Work out the finished part from the listing and answer in its coordinate system (mm). A direction names the side the tool comes from. Coordinates: 2 decimals unless noted, no trailing zeros. Order: outer loops, then holes, each group sorted by start corner. A loop starts at its lowest first (then second) coordinate and runs counter-clockwise, first axis right, second up. Notation, with made-up numbers: M -39,82 L -35,82 A23 cw -35,101 Z; hole C 46.5,1.5 d3. An arc over 180 degrees is marked long. Write item = value, one per line. Start each with the question number.
Q1. Find section C-C on x = 67.5. Give the vertices of the cut face in (y, z).
Q2. Find section A-A on x = -177. Give the vertices of the cut face in (y, z), and give its area (3 significant figures).
Q3. A tool of negligible diameter and unlimited length cuts with its end or side. For faces 4 (the flat face through (7, 0, 2)), 5 (the flat face through (0, 15, 147)), from which of +Z, -Z, +X, -X, +Y, -Y can it reach the whole face along a straight path? Write none if from no direction.
Q4. Determine the mould class of faces 1 (the flat face through (-500, 15, -13)), 2 (the cylindrical face through (7, 18.755, -171.923)), 3 (the flat face through (-253, 15, 145)) for opening direction Z: released by +Z, released by -Z, zero draft, split by the parting line, or undercut.
Q5. Find section B-B on y = 15. Give the vertices of the cut face in (x, z), and give its area (4 significant figures).
Q6. Straight lines are drawn through the part: line 1 along Z through (x, y) = (271, 19.5); line 2 along Z through (x, y) = (-10, 13.5); line 3 along Z through (x, y) = (262.5, 6). For each, find the intervals that lie inside material, in ascending order.
Q7. Each of these flat-tipped pins is pushed along its axis until it touches: P1, Ø12, axis at x = -247, y = 12, coming from the +Z side; P2, Ø12, axis at x = -304, y = 8, coming from the -Z side. Where does it stop, or does it pass through?
```python
from build123d import *

# Parameters (mm, degrees)
SKETCH1_W           = 1000
SKETCH1_H           = 290
BOSS_EXTRUDE1_DEPTH = 30
SKETCH2_R           = 15
SKETCH2_R_2         = 12.5
BOSS_EXTRUDE2_DEPTH = 500
SKETCH3_R           = 15
SKETCH3_R_2         = 12.5
BOSS_EXTRUDE3_DEPTH = 1000


with BuildPart() as part:
    # Sketch1 → Boss-Extrude1 (new body)
    with BuildSketch(Plane(origin=(0, 0, 0), x_dir=(1, 0, 0), z_dir=(0, 1, 0))):
        Rectangle(SKETCH1_W, SKETCH1_H)
    extrude(amount=BOSS_EXTRUDE1_DEPTH)

    # Sketch2 → Boss-Extrude2 (add)
    with BuildSketch(Plane(origin=(500, 0, 0), x_dir=(0, 0, -1), z_dir=(1, 0, 0))):
        with BuildLine():
            Line((-145, 30), (-160, 30))
            ThreePointArc((-160, 30), (-149.393398282, 25.606601718), (-145, 15))
            Line((-145, 15), (-145, 30))
        make_face()
        with BuildLine():
            Line((-145, 0), (-145, 15))
            ThreePointArc((-145, 15), (-149.393398282, 4.393398282), (-160, 0))
            Line((-160, 0), (-145, 0))
        make_face()
        with Locations((-160, 15)):
            Circle(SKETCH2_R)
        with Locations((-160, 15)):
            Circle(SKETCH2_R_2, mode=Mode.SUBTRACT)
    extrude(amount=-BOSS_EXTRUDE2_DEPTH)

    # Sketch3 → Boss-Extrude3 (add)
    with BuildSketch(Plane(origin=(500, 0, 0), x_dir=(0, 0, -1), z_dir=(1, 0, 0))):
        with BuildLine():
            ThreePointArc((145, 15), (149.393398282, 25.606601718), (160, 30))
            Line((160, 30), (145, 30))
            Line((145, 30), (145, 15))
        make_face()
        with Locations((160, 15)):
            Circle(SKETCH3_R)
        with Locations((160, 15)):
            Circle(SKETCH3_R_2, mode=Mode.SUBTRACT)
        with BuildLine():
            ThreePointArc((160, 0), (149.393398282, 4.393398282), (145, 15))
            Line((145, 15), (145, 0))
            Line((145, 0), (160, 0))
        make_face()
    extrude(amount=-BOSS_EXTRUDE3_DEPTH)


solid = part.part
```
Findings below:
q1.outline = M 0,-160 A15 ccw 30,-160 L 30,160 A15 ccw 0,160 Z; hole C 15,-160 d25; hole C 15,160 d25
q2.outline = M 0,-160 A15 ccw 30,-160 L 30,145 L 0,145 Z; hole C 15,-160 d25
q2.area = 9,010 mm^2
q3.face_4 = +Z, -Z, +X, -X, -Y
q3.face_5 = +Z, -X, +Y, -Y
q4.face_1 = zero draft
q4.face_2 = undercut
q4.face_3 = released by +Z
q5.outline = M -500,-175 L 500,-175 L 500,-172.5 L -500,-172.5 Z; M -500,-147.5 L 500,-147.5 L 500,147.5 L 0,147.5 L 0,145 L -500,145 Z; M 0,172.5 L 500,172.5 L 500,175 L 0,175 Z
q5.area = 297,500 mm^2
q6.line_1 = -174.31 to -171.66, -148.34 to 148.34, 171.66 to 174.31
q6.line_2 = -174.92 to -172.41, -147.59 to 145
q6.line_3 = -172 to -168.67, -151.33 to 151.33, 168.67 to 172
q7.P1 = 145
q7.P2 = -174.97
